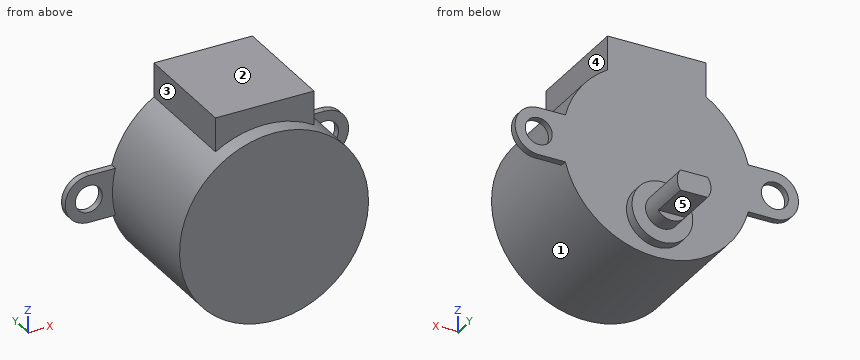
```python
from build123d import *

# Parameters (mm, degrees)
SKETCH_1_R          = 14
EXTRUDE_1_DEPTH     = 19
SKETCH_2_R          = 4.5
EXTRUDE_2_DEPTH     = 1.5
SKETCH_3_R          = 2.5
EXTRUDE_3_DEPTH     = 8.5
CUT_EXTRUDE_START   = -6
CUT_EXTRUDE_1_DEPTH = 6
EXTRUDE_START       = -1
SKETCH_5_R          = 2
EXTRUDE_4_DEPTH     = 1
EXTRUDE_START_2     = -16.5
EXTRUDE_5_DEPTH     = 16.5


with BuildPart() as part:
    # Эскиз1 → Бобышка-Вытянуть1 (new body)
    with BuildSketch(Plane(origin=(0, 0, 0), x_dir=(1, 0, 0), z_dir=(0, 1, 0))):
        with Locations(Location((0, 0, 0), (0, 0, 270))):
            Circle(SKETCH_1_R)
    extrude(amount=EXTRUDE_1_DEPTH)

    # Эскиз2 → Бобышка-Вытянуть2 (add)
    with BuildSketch(Plane(origin=(0, 19, 0), x_dir=(1, 0, 0), z_dir=(0, 1, 0))):
        with Locations(Location((0, 8, 0), (0, 0, 270))):
            Circle(SKETCH_2_R)
    extrude(amount=EXTRUDE_2_DEPTH)

    # Эскиз3 → Бобышка-Вытянуть3 (add)
    with BuildSketch(Plane(origin=(0, 20.5, 0), x_dir=(1, 0, 0), z_dir=(0, 1, 0))):
        with Locations(Location((0, 8, 0), (0, 0, 270))):
            Circle(SKETCH_3_R)
    extrude(amount=EXTRUDE_3_DEPTH)

    # Эскиз4 → Вырез-Вытянуть1 (cut)
    with BuildSketch(Plane(origin=(0, 29, 0), x_dir=(1, 0, 0), z_dir=(0, 1, 0)).offset(CUT_EXTRUDE_START)):
        with BuildLine():
            Line((-2, 9.5), (2, 9.5))
            ThreePointArc((2, 9.5), (0, 10.5), (-2, 9.5))
        make_face()
        with BuildLine():
            Line((-2, 6.5), (2, 6.5))
            ThreePointArc((2, 6.5), (0, 5.5), (-2, 6.5))
        make_face()
    extrude(amount=CUT_EXTRUDE_1_DEPTH, mode=Mode.SUBTRACT)

    # Эскиз5 → Бобышка-Вытянуть4 (add)
    # profile 1 of 2: a face of its own
    with BuildSketch(Plane(origin=(0, 19, 0), x_dir=(1, 0, 0), z_dir=(0, 1, 0)).offset(EXTRUDE_START)):
        with BuildLine():
            Line((-17.5, 3.5), (-13.555441712, 3.5))
            ThreePointArc((-13.555441712, 3.5), (-14, 0), (-13.555441712, -3.5))
            Line((-13.555441712, -3.5), (-17.5, -3.5))
            ThreePointArc((-17.5, -3.5), (-21, 0), (-17.5, 3.5))
        make_face()
        with Locations(Location((-17.5, 0, 0), (0, 0, 270))):
            Circle(SKETCH_5_R, mode=Mode.SUBTRACT)
    # profile 2 of 2: a face of its own
    with BuildSketch(Plane(origin=(0, 19, 0), x_dir=(1, 0, 0), z_dir=(0, 1, 0)).offset(EXTRUDE_START)):
        with BuildLine():
            Line((17.5, 3.5), (13.555441712, 3.5))
            ThreePointArc((13.555441712, 3.5), (14, 0), (13.555441712, -3.5))
            Line((13.555441712, -3.5), (17.5, -3.5))
            ThreePointArc((17.5, -3.5), (21, 0), (17.5, 3.5))
        make_face()
        with Locations(Location((17.5, 0, 0), (0, 0, 90))):
            Circle(SKETCH_5_R, mode=Mode.SUBTRACT)
    extrude(amount=EXTRUDE_4_DEPTH)

    # Эскиз6 → Бобышка-Вытянуть5 (add)
    with BuildSketch(Plane(origin=(0, 19, 0), x_dir=(1, 0, 0), z_dir=(0, 1, 0)).offset(EXTRUDE_START_2)):
        with BuildLine():
            Line((7.3, -17), (-7.3, -17))
            Line((-7.3, -17), (-7.3, -11.94612908))
            ThreePointArc((-7.3, -11.94612908), (0, -14), (7.3, -11.94612908))
            Line((7.3, -11.94612908), (7.3, -17))
        make_face()
    extrude(amount=EXTRUDE_5_DEPTH)


solid = part.part
```
Part model, mm, in its own coordinate system. Face numbers are marked on the shaded views. A direction names the side the tool comes from. Coordinates: 2 decimals unless noted, no trailing zeros. Write each loop counter-clockwise with the first axis right and the second up, starting at its lowest first coordinate (ties: lowest second). Pieces come first, ordered by that corner, then holes.
Item 1: Pin check, flat tips, straight feed: pin 1 (12 mm diameter, centred on x = -1, z = 4, fed in from +Y); pin 2 (4 mm diameter, centred on y = 7, z = 14.5, fed in from +X); pin 3 (4.5 mm diameter, centred on x = 0.5, y = 26, fed in from -Z); pin 4 (3 mm diameter, centred on x = -17.5, z = 0, fed in from -Y). Stop position of each tip, or through.
Item 2: Slice it at A-A (z = 0). Write the cut outline in (x, y).
Item 3: Slice it at C-C (y = 8). Write the cut outline in (x, z), and give its area (3 significant figures).
Item 4: Slice it at D-D (z = -6). Write the cut outline in (x, y).
Item 5: Which spindle directions (+Z, -Z, +X, -X, +Y, -Y) get a long thin tool onto all of the face, cutting with end or side? Do the marked faces 1, 2, 3, 4 and 5. Say none if no direction does.
Item 6: Slice it at B-B (x = -18). Write the cut outline in (y, z), and give its area (3 significant figures).
Item 7: Probe line 1 (X direction, y = 18.75, z = 0); line 2 (Z direction, x = 17.5, y = 18.4); line 3 (Y direction, x = 11.5, z = -2). List the from-to ranges inside material, lowest first.
Results found:
1. pin 1: stops at y = 19
1. pin 2: stops at x = 7.3
1. pin 3: stops at z = -9.5
1. pin 4: passes through
2. outline: (-21, 18) - (-19.5, 18) - (-19.5, 19) - (-21, 19) - close; (-15.5, 18) - (-14, 18) - (-14, 0) - (14, 0) - (14, 18) - (15.5, 18) - (15.5, 19) - (-15.5, 19) - close; (19.5, 18) - (21, 18) - (21, 19) - (19.5, 19) - close
3. outline: (-7.3, 11.95) arc R14 ccw (long way) to (7.3, 11.95) - (7.3, 17) - (-7.3, 17) - close
3. area: 669 mm2
4. outline: (-12.65, 0) - (12.65, 0) - (12.65, 19) - (4.03, 19) - (4.03, 20.5) - (1.5, 20.5) - (1.5, 23) - (-1.5, 23) - (-1.5, 20.5) - (-4.03, 20.5) - (-4.03, 19) - (-12.65, 19) - close
5. face 1: -Y
5. face 2: +Z, +X, -X, +Y, -Y
5. face 3: +Z, -X, +Y, -Y
5. face 4: +Z, +X, +Y, -Y
5. face 5: -Z, +X, -X, +Y
6. outline: (18, -3.46) - (19, -3.46) - (19, -1.94) - (18, -1.94) - close; (18, 1.94) - (19, 1.94) - (19, 3.46) - (18, 3.46) - close
6. area: 3.06 mm2
7. line 1: x = -21 to -19.5, -15.5 to 15.5, 19.5 to 21
7. line 2: z = -3.5 to -2, 2 to 3.5
7. line 3: y = 0 to 19
